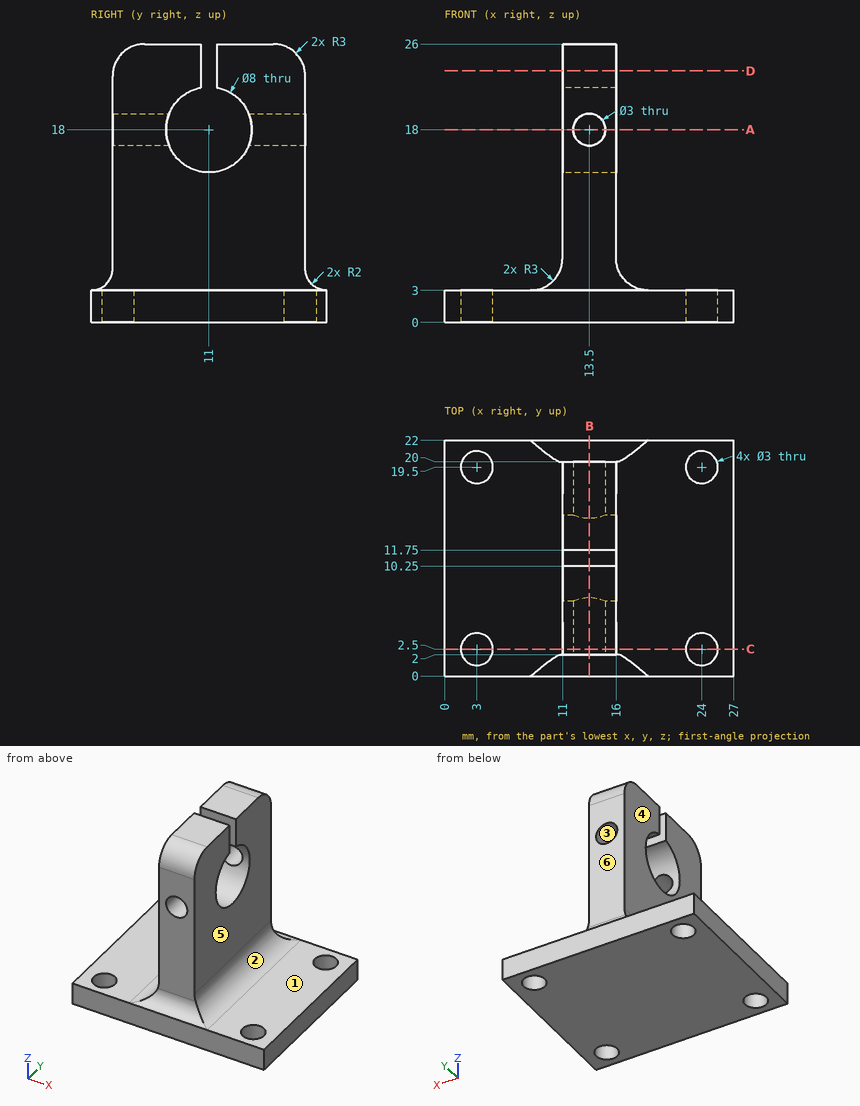
Part print with two shaded views. Sizes in mm from the minimum x, y, z corner. A direction names the side the tool comes from. Round coordinates to 2 decimals unless told otherwise and drop trailing zeros. Order: outer loops, then holes, each group sorted by start corner. A loop starts at its lowest first (then second) coordinate and runs counter-clockwise, first axis right, second up. Notation, with made-up numbers: M 79.25,49 L 108.25,49 A19 cw 108.25,71 Z; hole C -14.5,71.5 d7. An arc over 180 degrees is marked long. Put each result on its own line as item: value. Start each with the question number.
1. Slice it at C-C on y = 2.5. List the corners of the cut face in (x, z).
2. Slice it at B-B on x = 13.5. State how many separate pieces and enclosed holes the cut face has, then the cut area to 3 significant figures.
3. Slice it at D-D on z = 23.5. List the corners of the cut face in (x, y), then the cut area to 3 significant figures.
4. Tool access for the marked faces 4, 5 and 6: list every direction of +Z, -Z, +X, -X, +Y, -Y with a clear straight run to the whole face (end or side of a thin tool).
5. Drop flat-ended pins along their axis: pin 1 (1.5 mm diameter, centred on x = 18, y = 3, fed in from +Z); pin 2 (5 mm diameter, centred on x = 3, y = 19.5, fed in from +Z); pin 3 (2.5 mm diameter, centred on x = 24, y = 19.5, fed in from +Z); pin 4 (4.5 mm diameter, centred on x = 14, z = 17.5, fed in from -Y). Give the stop position or say it passes through.
6. Slice it at A-A on z = 18. List the corners of the cut face in (x, y).
7. Drill centre lines: probe 1 along Y at (x, z) = (3, 2.3); probe 2 along Z at (x, y) = (13.5, 5.55); probe 3 along Z at (x, y) = (5.25, 21.25). Where is each one in solid material? Low to high. Write a range as [from, to].
8. Two-plate mould, pull along X, no slides. Class the marked faces 1, 2 and 3: +X half, -X half, draft (parallel to the pull), parting line (faces both ways), or undercut.
Findings:
1. outline: M 0,0 L 1.5,0 L 1.5,3 L 0,3 Z; M 4.5,0 L 22.5,0 L 22.5,3 L 19,3 A3 cw 16,6 L 16,24.66 L 11,24.66 L 11,6 A3 cw 8,3 L 4.5,3 Z; M 25.5,0 L 27,0 L 27,3 L 25.5,3 Z; hole C 13.5,18 d3
2. separate pieces: 3
2. enclosed holes: 0
2. area: 391 mm2
3. outline: M 11,2.04 L 16,2.04 L 16,10.25 L 11,10.25 Z; M 11,11.75 L 16,11.75 L 16,19.96 L 11,19.96 Z
3. area: 82.1 mm2
4. face 4: +Z, -X, +Y, -Y
4. face 5: +Z, +X, +Y, -Y
4. face 6: +Z, +X, -X, +Y
5. pin 1: z = 3.56
5. pin 2: z = 3
5. pin 3: through
5. pin 4: y = 2
6. outline: M 11,2 L 12,2 L 12,7 L 11,7 Z; M 11,15 L 12,15 L 12,20 L 11,20 Z; M 15,2 L 16,2 L 16,7 L 15,7 Z; M 15,15 L 16,15 L 16,20 L 15,20 Z
7. probe 1: [0, 1], [4, 18], [21, 22]
7. probe 2: [0, 16.5], [19.5, 26]
7. probe 3: [0, 3]
8. face 1: draft
8. face 2: +X half
8. face 3: undercut
